from build123d import *

# Parameters (mm, degrees)
ESQUISSE1_W             = 20
ESQUISSE1_H             = 20
BOSS_EXTRU_1_DEPTH      = 120
ESQUISSE2_W             = 1.2
ESQUISSE2_H             = 5.5
ESQUISSE2_W_2           = 5.5
ESQUISSE2_H_2           = 1.2
ENL_V_MAT_EXTRU_1_DEPTH = 121
ENL_V_MAT_EXTRU_2_DEPTH = 121
ESQUISSE4_R             = 2.5
ENL_V_MAT_EXTRU_3_DEPTH = 121


with BuildPart() as part:
    # Esquisse1 → Boss.-Extru.1 (new body)
    with BuildSketch(Plane.XY):
        with Locations((-12.505109137, -9.909560068)):
            Rectangle(ESQUISSE1_W, ESQUISSE1_H)
    extrude(amount=BOSS_EXTRU_1_DEPTH)

    # Esquisse2 → Enlèv. mat.-Extru.1 (cut, through all)
    with BuildSketch(Plane.XY.offset(120)):
        with Locations((-21.905109137, -9.909560068)):
            Rectangle(ESQUISSE2_W, ESQUISSE2_H)
        with Locations((-12.505109137, -0.509560068)):
            Rectangle(ESQUISSE2_W_2, ESQUISSE2_H_2)
        with Locations((-3.105109137, -9.909560068)):
            Rectangle(ESQUISSE2_W, ESQUISSE2_H)
        with Locations((-12.505109137, -19.309560068)):
            Rectangle(ESQUISSE2_W_2, ESQUISSE2_H_2)
    extrude(amount=-ENL_V_MAT_EXTRU_1_DEPTH, mode=Mode.SUBTRACT)

    # Esquisse3 → Enlèv. mat.-Extru.2 (cut, through all)
    with BuildSketch(Plane.XY.offset(120)):
        Polygon((-21.305109137, -15.909560068), (-20.305109137, -15.909560068), (-17.305109137, -12.909560068), (-17.305109137, -6.909560068), (-20.305109137, -3.909560068), (-21.305109137, -3.909560068), align=None)
        Polygon((-18.505109137, -1.109560068), (-6.505109137, -1.109560068), (-6.505109137, -2.109560068), (-9.505109137, -5.109560068), (-15.505109137, -5.109560068), (-18.505109137, -2.109560068), align=None)
        Polygon((-3.705109137, -3.909560068), (-4.705109137, -3.909560068), (-7.705109137, -6.909560068), (-7.705109137, -12.909560068), (-4.705109137, -15.909560068), (-3.705109137, -15.909560068), align=None)
        Polygon((-6.505109137, -18.709560068), (-18.505109137, -18.709560068), (-18.505109137, -17.709560068), (-15.505109137, -14.709560068), (-9.505109137, -14.709560068), (-6.505109137, -17.709560068), align=None)
    extrude(amount=-ENL_V_MAT_EXTRU_2_DEPTH, mode=Mode.SUBTRACT)

    # Esquisse4 → Enlèv. mat.-Extru.3 (cut, through all)
    with BuildSketch(Plane.XY.offset(120)):
        with Locations((-12.505109137, -9.909560068)):
            Circle(ESQUISSE4_R)
    extrude(amount=-ENL_V_MAT_EXTRU_3_DEPTH, mode=Mode.SUBTRACT)


solid = part.part
Could you check a few things on this model? Use its own coordinates, in mm. A direction names the side the tool comes from. Give positions to 0.01 mm unless a question says otherwise; leave off trailing zeros. Order: outer loops, then holes, each group sorted by start corner. A loop starts at its lowest first (then second) coordinate and runs counter-clockwise, first axis right, second up.
1. Suppose I cut it at A-A (y = -11). List the corners of the cut face in (x, z) for me, plus the area to 3 significant figures.
2. I need wall thicknesses on L1, parallel to Y at x = -9.5, z = 25.5; L2, parallel to X at y = -1.75, z = 36; L3, parallel to X at y = -6.75, z = 34. Which ranges of each line are inside material? Lowest first, please.
3. For faces 5 (the flat face through (-18.784, -5.431, 60.84)), 6 (the flat face through (-19, -19.91, 59)), which set-ups out of +Z, -Z, +X, -X, +Y, -Y let a thin tool reach every point of the face, with its end or its side?
4. Suppose I cut it at B-B (x = -13.5). List the corners of the cut face in (y, z) for me, plus the area to 3 significant figures.
5. We'd pull the mould along Y, two halves only. Please class faces 1 (the flat face through (-8, -1.11, 61)), 2 (the flat face through (-15, -8, 0)), 3 (the flat face through (-19, 0.09, 59)), 4 (the flat face through (-6, -19.91, 59)): pulls with the +Y half, pulls with the -Y half, needs draft (parallel to the pull), parting line crosses it, or undercut.
6. Will these pins go through, and if not, where does the flat tip stop? P1, Ø3, axis at x = -12, y = -2.5, coming from the +Z side; P2, Ø3, axis at x = -11.5, z = 78, coming from the +Y side.
Solved:
1. outline: (-17.31, 0) - (-14.75, 0) - (-14.75, 120) - (-17.31, 120) - close; (-10.26, 0) - (-7.71, 0) - (-7.71, 120) - (-10.26, 120) - close
1. area: 612 mm2
2. L1: y = -19.91 to -18.71, -14.71 to -5.1, -1.11 to 0.09
2. L2: x = -22.51 to -18.51, -6.51 to -2.51
2. L3: x = -22.51 to -21.31, -17.46 to -7.55, -3.71 to -2.51
3. face 5: +Z, -Z
3. face 6: +Z, -Z, +X, -X, -Y
4. outline: (-14.71, 0) - (-12.2, 0) - (-12.2, 120) - (-14.71, 120) - close; (-7.62, 0) - (-5.11, 0) - (-5.11, 120) - (-7.62, 120) - close
4. area: 602 mm2
5. face 1: undercut
5. face 2: needs draft
5. face 3: pulls with the +Y half
5. face 4: pulls with the -Y half
6. P1: passes through
6. P2: stops at y = -5.11
